```python
from build123d import *
from OCP.BRepFilletAPI import BRepFilletAPI_MakeChamfer

# Parameters (mm, degrees)
BOSS_EXTRUDE1_DEPTH = 5
FILLET2_R           = 15
FILLET3_R           = 10
SHELL1_T            = -3.2
BOSS_EXTRUDE2_DEPTH = 5.2
CHAMFER1_SIZE       = 1
CHAMFER1_SIZE2      = 0.577350269
SKETCH2_R           = 8
CUT_EXTRUDE1_DEPTH  = 64.128614634
SKETCH3_R           = 6
CUT_EXTRUDE2_DEPTH  = 64.128614634


with BuildPart() as part:
    # Sketch1 → Boss-Extrude1 (new body)
    with BuildSketch(Plane(origin=(0, 0, 0), x_dir=(1, 0, 0), z_dir=(0, 1, 0))):
        with BuildLine():
            Line((17.5, 0), (-17.5, 0))
            Line((-17.5, 0), (-38, 30))
            Line((-38, 30), (-38, 40))
            ThreePointArc((-38, 40), (0, 50), (38, 40))
            Line((38, 40), (38, 30))
            Line((38, 30), (17.5, 0))
        make_face()
    extrude(amount=BOSS_EXTRUDE1_DEPTH)

    # Fillet2
    fillet2_edges = [part.edges().sort_by_distance(p)[0] for p in [
        (-38, 2.5, -40),
        (38, 2.5, -40),
    ]]
    fillet(fillet2_edges, radius=FILLET2_R)

    # Fillet3
    fillet3_edges = [part.edges().sort_by_distance(p)[0] for p in [
        (38, 2.5, -30),
        (-38, 2.5, -30),
    ]]
    fillet(fillet3_edges, radius=FILLET3_R)

    # Shell1
    shell1_openings = [part.faces().sort_by_distance(p)[0] for p in [
        (0, 0, -26.14204648),
    ]]
    offset(amount=SHELL1_T, openings=shell1_openings)

    # Sketch5 → Boss-Extrude2 (add)
    with BuildSketch(Plane.XZ.offset(-1.8)):
        with BuildLine():
            Line((15.810907243, -3.2), (-15.810907243, -3.2))
            Line((-15.810907243, -3.2), (-33.226375888, -28.686051676))
            ThreePointArc((-33.226375888, -28.686051676), (-34.377028804, -31.833866159), (-33.88430189, -35.148976767))
            ThreePointArc((-33.88430189, -35.148976767), (-31.269334859, -39.009074238), (-27.363344051, -41.554980927))
            ThreePointArc((-27.363344051, -41.554980927), (0, -46.8), (27.363344051, -41.554980927))
            ThreePointArc((27.363344051, -41.554980927), (31.269334859, -39.009074238), (33.88430189, -35.148976767))
            ThreePointArc((33.88430189, -35.148976767), (34.377028804, -31.833866159), (33.226375888, -28.686051676))
            Line((33.226375888, -28.686051676), (15.810907243, -3.2))
        make_face()
    extrude(amount=BOSS_EXTRUDE2_DEPTH)

    # Chamfer1: one chamfer whose edges measure the first distance from different faces: ONE call of the kernel's chamfer builder (chamfer() names one face for all edges)
    chamfer1_edges_1 = [part.edges().sort_by_distance(p)[0] for p in [
        (24.518641566, -3.4, -15.943025838),
    ]]
    chamfer1_side_1 = [part.faces().sort_by_distance(p)[0] for p in [
        (24.518641566, -1.7, -15.943025838),
    ]]
    chamfer1_edges_2 = [part.edges().sort_by_distance(p)[0] for p in [
        (0, -3.4, -3.2),
    ]]
    chamfer1_side_2 = [part.faces().sort_by_distance(p)[0] for p in [
        (0, -1.7, -3.2),
    ]]
    chamfer1_edges_3 = [part.edges().sort_by_distance(p)[0] for p in [
        (-24.518641566, -3.4, -15.943025838),
    ]]
    chamfer1_side_3 = [part.faces().sort_by_distance(p)[0] for p in [
        (-24.518641566, -1.7, -15.943025838),
    ]]
    chamfer1_edges_4 = [part.edges().sort_by_distance(p)[0] for p in [
        (-34.377028804, -3.4, -31.833866159),
    ]]
    chamfer1_side_4 = [part.faces().sort_by_distance(p)[0] for p in [
        (-34.377028804, -1.7, -31.833866159),
    ]]
    chamfer1_edges_5 = [part.edges().sort_by_distance(p)[0] for p in [
        (-31.269334859, -3.4, -39.009074238),
    ]]
    chamfer1_side_5 = [part.faces().sort_by_distance(p)[0] for p in [
        (-31.269334859, -1.7, -39.009074238),
    ]]
    chamfer1_edges_6 = [part.edges().sort_by_distance(p)[0] for p in [
        (0, -3.4, -46.8),
    ]]
    chamfer1_side_6 = [part.faces().sort_by_distance(p)[0] for p in [
        (0, -1.7, -46.8),
    ]]
    chamfer1_edges_7 = [part.edges().sort_by_distance(p)[0] for p in [
        (31.269334859, -3.4, -39.009074238),
    ]]
    chamfer1_side_7 = [part.faces().sort_by_distance(p)[0] for p in [
        (31.269334859, -1.7, -39.009074238),
    ]]
    chamfer1_edges_8 = [part.edges().sort_by_distance(p)[0] for p in [
        (34.377028804, -3.4, -31.833866159),
    ]]
    chamfer1_side_8 = [part.faces().sort_by_distance(p)[0] for p in [
        (34.377028804, -1.7, -31.833866159),
    ]]
    chamfer1 = BRepFilletAPI_MakeChamfer(part.part.solid().wrapped)
    for e in chamfer1_edges_1:
        chamfer1.Add(CHAMFER1_SIZE, CHAMFER1_SIZE2, e.wrapped, chamfer1_side_1[0].wrapped)  # the first distance lies on this face
    for e in chamfer1_edges_2:
        chamfer1.Add(CHAMFER1_SIZE, CHAMFER1_SIZE2, e.wrapped, chamfer1_side_2[0].wrapped)  # the first distance lies on this face
    for e in chamfer1_edges_3:
        chamfer1.Add(CHAMFER1_SIZE, CHAMFER1_SIZE2, e.wrapped, chamfer1_side_3[0].wrapped)  # the first distance lies on this face
    for e in chamfer1_edges_4:
        chamfer1.Add(CHAMFER1_SIZE, CHAMFER1_SIZE2, e.wrapped, chamfer1_side_4[0].wrapped)  # the first distance lies on this face
    for e in chamfer1_edges_5:
        chamfer1.Add(CHAMFER1_SIZE, CHAMFER1_SIZE2, e.wrapped, chamfer1_side_5[0].wrapped)  # the first distance lies on this face
    for e in chamfer1_edges_6:
        chamfer1.Add(CHAMFER1_SIZE, CHAMFER1_SIZE2, e.wrapped, chamfer1_side_6[0].wrapped)  # the first distance lies on this face
    for e in chamfer1_edges_7:
        chamfer1.Add(CHAMFER1_SIZE, CHAMFER1_SIZE2, e.wrapped, chamfer1_side_7[0].wrapped)  # the first distance lies on this face
    for e in chamfer1_edges_8:
        chamfer1.Add(CHAMFER1_SIZE, CHAMFER1_SIZE2, e.wrapped, chamfer1_side_8[0].wrapped)  # the first distance lies on this face
    add(Compound.cast(chamfer1.Shape()), mode=Mode.REPLACE)

    # Sketch2 → Cut-Extrude1 (cut, through all)
    with BuildSketch(Plane(origin=(0, 5, 0), x_dir=(1, 0, 0), z_dir=(0, 1, 0))):
        with Locations(Location((0, 12, 0), (0, 0, 270))):
            Circle(SKETCH2_R)
    extrude(amount=-CUT_EXTRUDE1_DEPTH, mode=Mode.SUBTRACT)

    # Sketch3 → Cut-Extrude2 (cut, through all)
    with BuildSketch(Plane(origin=(0, 5, 0), x_dir=(1, 0, 0), z_dir=(0, 1, 0))):
        with Locations(Location((-17, 28, 0), (0, 0, 270))):
            Circle(SKETCH3_R)
        with Locations(Location((18, 32, 0), (0, 0, 270))):
            Circle(SKETCH3_R)
    extrude(amount=-CUT_EXTRUDE2_DEPTH, mode=Mode.SUBTRACT)


solid = part.part
```
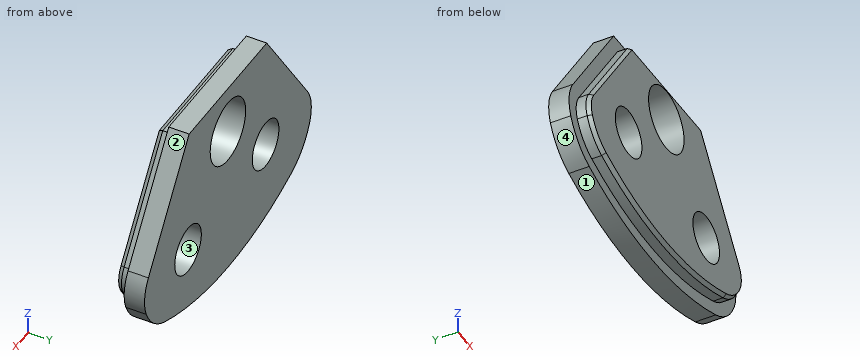
Geometry check sheet. Reference: the model listing, model coordinates, mm. Face numbers are marked on the shaded views. Round coordinates to 2 decimals unless told otherwise and drop trailing zeros. Order: outer loops, then holes, each group sorted by start corner. A loop starts at its lowest first (then second) coordinate and runs counter-clockwise, first axis right, second up. Notation, with made-up numbers: (66, 13) - (110, 13) arc R31 cw to (110, 41) - close; hole circle Ø10 at (-19.75, 58). An arc over 180 degrees is marked (long way). Use a Markdown table: item, result. Add a question column.
1) Section check B-B (x = 0). Record the cut outline in (y, z).
2) Mould release check, pull along X, two halves, no side actions. Record for the marked faces 1, 2, 3 and 4: released by +X, released by -X, zero draft, split by the parting line, or undercut.
3) Section check A-A (y = -1.5). Record the cut outline in (x, z).
4) Section check D-D (z = -32). Count the separate pieces of the cut face and the enclosed holes in it, then the cut area to 3 significant figures.
5) Gauge pin test, flat ends, axial feed: P1, Ø7, axis at x = 18, z = -32, coming from the -Y side; P2, Ø4, axis at x = 13, y = -2.5, coming from the +Z side; P3, Ø1, axis at x = 28, y = 4, coming from the -Z side; P4, Ø1, axis at y = 1, z = -40.5, coming from the -X side. Record the tip position at first contact, or that the pin passes through.
6) Thickness scan on line 1 along X through (y, z) = (-1.5, -28); line 2 along Y through (x, z) = (13.5, -46.5); line 3 along X through (y, z) = (2.5, -12). Record the ranges inside material, lowest first.
7) Section check C-C (z = -5). Record the cut outline in (x, y).
Established:
| question | item | result |
|---|---|---|
| 1 | outline | (-3.4, -46.22) - (-2.4, -46.8) - (0, -46.8) - (0, -50) - (5, -50) - (5, -20) - (-3.4, -20) - close; (-3.4, -4) - (5, -4) - (5, 0) - (0, 0) - (0, -3.2) - (-2.4, -3.2) - (-3.4, -3.78) - close |
| 2 | face 1 | split by the parting line |
| 2 | face 2 | released by +X |
| 2 | face 3 | undercut |
| 2 | face 4 | released by -X |
| 3 | outline | (-33.88, -35.15) arc R11.8 ccw to (-27.36, -41.55) arc R74 ccw to (27.36, -41.55) arc R11.8 ccw to (33.88, -35.15) arc R6.8 ccw to (33.23, -28.69) - (15.81, -3.2) - (-15.81, -3.2) - (-33.23, -28.69) arc R6.8 ccw to start; hole circle Ø12 at (-17, -28); hole circle Ø16 at (0, -12); hole circle Ø12 at (18, -32) |
| 4 | separate pieces | 3 |
| 4 | enclosed holes | 0 |
| 4 | area | 433 mm2 |
| 5 | P1 | through |
| 5 | P2 | z = -3.2 |
| 5 | P3 | z = -44.94 |
| 5 | P4 | x = -34.68 |
| 6 | line 1 | -32.76 to -23, -11 to 13.53, 22.47 to 32.76 |
| 6 | line 2 | 0 to 5 |
| 6 | line 3 | -25.7 to -8, 8 to 25.7 |
| 7 | outline | (-20.92, 0) - (-17.04, 0) - (-17.04, -2.4) - (-16.34, -3.4) - (-3.87, -3.4) - (-3.87, 5) - (-20.92, 5) - close; (3.87, -3.4) - (16.34, -3.4) - (17.04, -2.4) - (17.04, 0) - (20.92, 0) - (20.92, 5) - (3.87, 5) - close |
